Source: CAD feature listing. Evaluate the final solid. Frame: model axes, mm. A direction names the side the tool comes from. Coordinates: 2 decimals unless noted, no trailing zeros. Loops run counter-clockwise (first coordinate to the right, second up) from the corner with the lowest first, then second, coordinate; pieces in that order, holes last. Notation, with made-up numbers: (-12, 78) -> (20, 78) arc R21 cw to (20, 90) -> close; hole circle Ø3 at (62.25, 18.5). An arc over 180 degrees is marked (long way). Answer as CSV lines item,"result".
from build123d import *

# Parameters (mm, degrees)
SKETCH_1_W         = 6.08
SKETCH_1_H         = 6.83
EXTRUDE_1_DEPTH    = 4.12
SKETCH_2_R         = 2.35
EXTRUDE_2_DEPTH    = 0.1
DOME_1_FACE_RADIUS = 2.35
DOME_1_HEIGHT      = 1.45


with BuildPart() as part:
    # 草图1 → 拉伸1 (new body)
    with BuildSketch(Plane.XY):
        Rectangle(SKETCH_1_W, SKETCH_1_H)
    extrude(amount=EXTRUDE_1_DEPTH)

    # 草图2 → 拉伸2 (add)
    with BuildSketch(Plane(origin=(0, 0, 0), x_dir=(-1, 0, 0), z_dir=(0, 0, -1))):
        with Locations(Location((0, 0.565, 0), (0, 0, 180))):
            Circle(SKETCH_2_R)
    extrude(amount=EXTRUDE_2_DEPTH)

    # 圆顶1: a dome of height H over a round flat face of radius A is a cap of a sphere of radius (A * A + H * H) / (2 * H)
    dome_1_r = (DOME_1_FACE_RADIUS * DOME_1_FACE_RADIUS + DOME_1_HEIGHT * DOME_1_HEIGHT) / (2 * DOME_1_HEIGHT)
    dome_1_base = Plane((0, 0.565, -0.1), z_dir=(0, 0, -1))
    with Locations(dome_1_base.offset(DOME_1_HEIGHT - dome_1_r)):
        dome_1_ball = Sphere(dome_1_r, mode=Mode.PRIVATE)
    add(split(dome_1_ball, bisect_by=dome_1_base, keep=Keep.TOP, mode=Mode.PRIVATE))


solid = part.part
(1) Cut plane B-B (y = -0.5). Return the cut outline in (x, z).
Computed values:
outline,"(-3.04, 0) -> (-2.09, 0) -> (-2.09, -0.1) arc R2.4 ccw to (2.09, -0.1) -> (2.09, 0) -> (3.04, 0) -> (3.04, 4.12) -> (-3.04, 4.12) -> close"
(2) Access query for faces 1 (the flat face through (0, -2, 0)), 2 (the flat face through (3.04, 0, 2)). Directions: +Z, -Z, +X, -X, +Y, -Y. A direction counts if a zero-diameter tool reaches every point of the face in a straight line with its end or side. Return the directions, or none.
Computed values:
face 1,"-Z"
face 2,"+Z, -Z, +X, +Y, -Y"
(3) Cut plane C-C (z = -0.3). Return the cut outline in (x, y) (3 decimals).
Computed values:
outline,"circle Ø4.477 at (0, 0.565)"
(4) Cut plane A-A (x = 0). Return the cut outline in (y, z) (3 decimals), then the cut area to 3 significant figures.
Computed values:
outline,"(-3.415, 0) -> (-1.785, 0) -> (-1.785, -0.1) arc R2.629 ccw to (2.915, -0.1) -> (2.915, 0) -> (3.415, 0) -> (3.415, 4.12) -> (-3.415, 4.12) -> close"
area,"33.5 mm^2"
(5) Material intervals for L1, parallel to Z at x = -2.5, y = -2; L2, parallel to X at y = -1, z = -0.55; L3, parallel to Z at x = 0, y = -0.5, sorted ascending. Write a range as [from, to].
Computed values:
L1,"[0, 4.12]"
L2,"[-1.35, 1.35]"
L3,"[-1.32, 4.12]"
(6) Cut plane D-D (y = -2). Return the cut outline in (x, z).
Computed values:
outline,"(-3.04, 0) -> (3.04, 0) -> (3.04, 4.12) -> (-3.04, 4.12) -> close"
(7) Pin query (flat end, axial travel): pin 1 Ø1.5 at (x, y) = (-1, -1.5) entering from -Z. Return the tip coordinate at first contact, or that it passes through.
Computed values:
pin 1,"z = -1.05"
